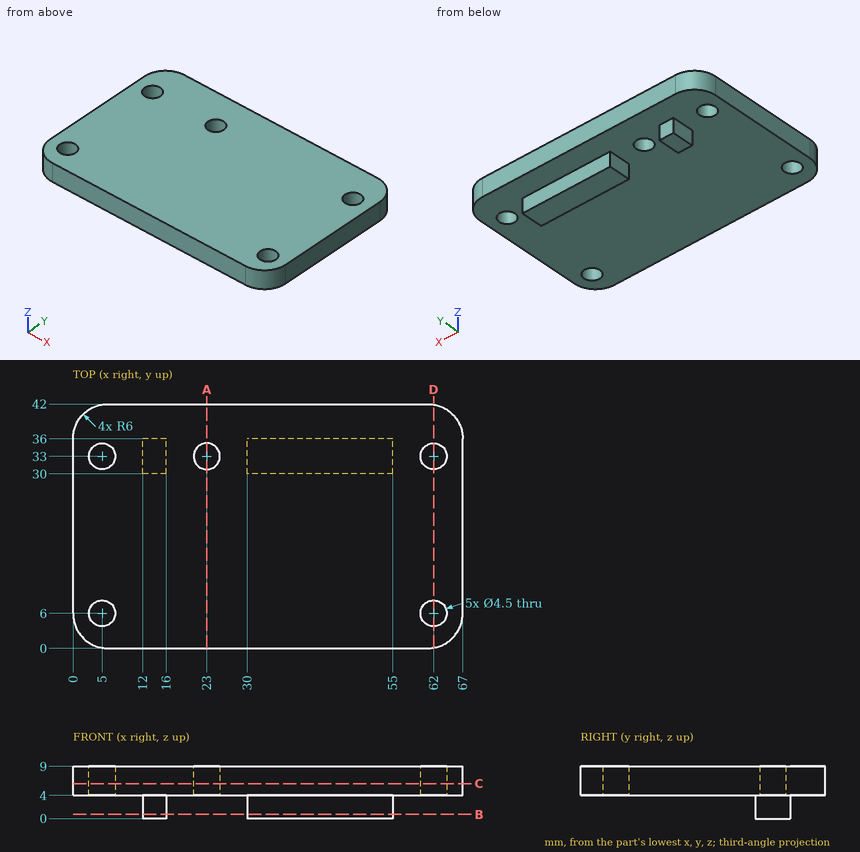
The figure shows three views and two pictorial views of one solid part (mm, origin at its lowest corner). Answer the questions. Round coordinates to 2 decimals unless told otherwise and drop trailing zeros. Order: outer loops, then holes, each group sorted by start corner. A loop starts at its lowest first (then second) coordinate and runs counter-clockwise, first axis right, second up. Notation, with made-up numbers: (55, -37.5) -> (78, -37.5) arc R18 ccw to (78, -9.5) -> close; hole circle Ø11 at (-31, 77.5). An arc over 180 degrees is marked (long way). Put each result on its own line as item: value.
Q1. Consider line 1 along Y through (x, z) = (62, 5.4); line 2 along X through (y, z) = (8, 5); line 3 along Z through (x, y) = (51.5, 17). Determine where each line is inside the solid, lowest interval first.
Results list:
line 1: 0.08 to 3.75, 8.25 to 30.75, 35.25 to 41.92
line 2: 0 to 3.97, 6.03 to 60.97, 63.03 to 67
line 3: 4 to 9
Q2. Each of these flat-tipped pins is pushed along its axis until it touches: P1, Ø3, axis at y = 33.5, z = 1.5, coming from the -X side; P2, Ø2, axis at y = 33, z = 1.5, coming from the +X side; P3, Ø6, axis at x = 62, y = 33, coming from the -Z side. Where does it stop, or does it pass through?
Results list:
P1: x = 12
P2: x = 55
P3: z = 4
Q3. Section C-C, the plane z = 6 is taken. Write down the section's boundary in (x, y).
Results list:
outline: (0, 6) arc R6 ccw to (6, 0) -> (61, 0) arc R6 ccw to (67, 6) -> (67, 36) arc R6 ccw to (61, 42) -> (6, 42) arc R6 ccw to (0, 36) -> close; hole circle Ø4.5 at (5, 6); hole circle Ø4.5 at (5, 33); hole circle Ø4.5 at (23, 33); hole circle Ø4.5 at (62, 6); hole circle Ø4.5 at (62, 33)
Q4. Section A-A, the plane x = 23 is taken. Write down the section's boundary in (y, z), and give its area (4 significant figures).
Results list:
outline: (0, 4) -> (30.75, 4) -> (30.75, 9) -> (0, 9) -> close; (35.25, 4) -> (42, 4) -> (42, 9) -> (35.25, 9) -> close
area: 187.5 mm^2
Q5. Section B-B, the plane z = 0.75 is taken. Write down the section's boundary in (x, y), and give its area (3 significant figures).
Results list:
outline: (12, 30) -> (16, 30) -> (16, 36) -> (12, 36) -> close; (30, 30) -> (55, 30) -> (55, 36) -> (30, 36) -> close
area: 174 mm^2
Q6. Section D-D, the plane x = 62 is taken. Write down the section's boundary in (y, z).
Results list:
outline: (0.08, 4) -> (3.75, 4) -> (3.75, 9) -> (0.08, 9) -> close; (8.25, 4) -> (30.75, 4) -> (30.75, 9) -> (8.25, 9) -> close; (35.25, 4) -> (41.92, 4) -> (41.92, 9) -> (35.25, 9) -> close
